The listing builds one solid part. Answer for the finished solid, in the listing's coordinates (mm). Face numbers are marked on the shaded views. A direction names the side the tool comes from. Give positions to 0.01 mm unless a question says otherwise; leave off trailing zeros. Order: outer loops, then holes, each group sorted by start corner. A loop starts at its lowest first (then second) coordinate and runs counter-clockwise, first axis right, second up. Notation, with made-up numbers: (-8.5, 35) - (6.5, 35) arc R34 ccw to (6.5, 66) - close; hole circle Ø3 at (37.25, 4.5). An arc over 180 degrees is marked (long way). Use a Markdown table: item, result. Add a question column.
1) Find section B-B, the plane z = 15. Determine the outline of the cut face in (x, y), plus the area to 3 significant figures.
2) For the marked faces 1 and 2, determine the directions among +Z, -Z, +X, -X, +Y, -Y from which every point of the face is accessible in a straight line to the end or side of a thin tool.
3) Find section C-C, the plane z = 0. Determine the outline of the cut face in (x, y), plus the area to 3 significant figures.
4) Find section D-D, the plane x = -2. Determine the outline of the cut face in (y, z).
5) Straight lines are drawn through the part: line 1 (X direction, y = 3.1, z = 0); line 2 (Z direction, x = -7, y = 3.55); line 3 (Y direction, x = -25, z = -9). For each, find the intervals that lie inside material, in ascending order.
6) The mould has two halves that part along X. Classify the marked faces 3 and 4: released by +X, released by -X, zero draft, split by the parting line, or undercut.
7) A flat-ended cylindrical pin translates along its axis: pin 1 (6 mm diameter, centred on x = 22.5, z = -0.5, fed in from +Y). Find the tip coordinate at first contact, or state that the pin passes through.
8) Find section A-A, the plane x = 15. Determine the outline of the cut face in (y, z), plus the area to 3 significant figures.
from build123d import *

# Parameters (mm, degrees)
CROQUIS1_W              = 70
CROQUIS1_H              = 40
SALIENTE_EXTRUIR1_DEPTH = 2
CROQUIS2_R              = 16
CROQUIS2_R_2            = 14
CROQUIS2_R_3            = 9.98
CROQUIS2_R_4            = 10
CROQUIS2_R_5            = 7.75
CROQUIS2_R_6            = 4.98
SALIENTE_EXTRUIR2_DEPTH = 2


with BuildPart() as part:
    # Croquis1 → Saliente-Extruir1 (new body)
    with BuildSketch(Plane(origin=(0, 0, 0), x_dir=(1, 0, 0), z_dir=(0, 1, 0))):
        Rectangle(CROQUIS1_W, CROQUIS1_H)
    extrude(amount=SALIENTE_EXTRUIR1_DEPTH)

    # Croquis2 → Saliente-Extruir2 (add)
    # profile 1 of 4: a face of its own
    with BuildSketch(Plane(origin=(0, 2, 0), x_dir=(1, 0, 0), z_dir=(0, 1, 0))):
        with Locations(Location((-15, 0, 0), (0, 0, 90))):
            Circle(CROQUIS2_R)
        with Locations(Location((-15, 0, 0), (0, 0, 270))):
            Circle(CROQUIS2_R_2, mode=Mode.SUBTRACT)
    # profile 2 of 4: a face of its own
    with BuildSketch(Plane(origin=(0, 2, 0), x_dir=(1, 0, 0), z_dir=(0, 1, 0))):
        with Locations(Location((-15, 0, 0), (0, 0, 90))):
            Circle(CROQUIS2_R_3)
    # profile 3 of 4: a face of its own
    with BuildSketch(Plane(origin=(0, 2, 0), x_dir=(1, 0, 0), z_dir=(0, 1, 0))):
        with Locations(Location((15, 0, 0), (0, 0, 90))):
            Circle(CROQUIS2_R_4)
        with Locations(Location((15, 0, 0), (0, 0, 270))):
            Circle(CROQUIS2_R_5, mode=Mode.SUBTRACT)
    # profile 4 of 4: a face of its own
    with BuildSketch(Plane(origin=(0, 2, 0), x_dir=(1, 0, 0), z_dir=(0, 1, 0))):
        with Locations(Location((15, 0, 0), (0, 0, 90))):
            Circle(CROQUIS2_R_6)
    extrude(amount=SALIENTE_EXTRUIR2_DEPTH)


solid = part.part
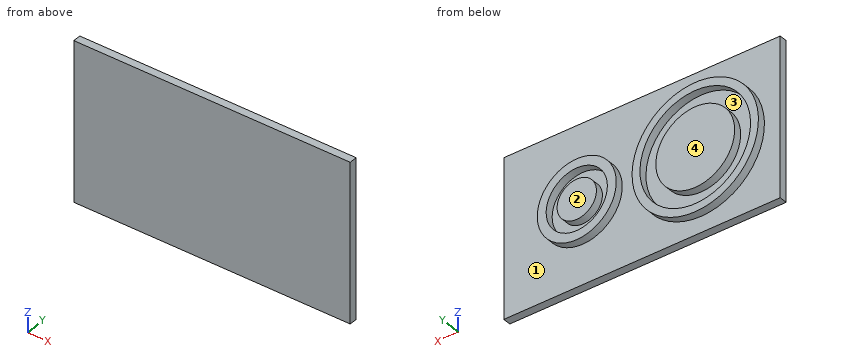
The answers:
| question | item | result |
|---|---|---|
| 1 | outline | (-35, 0) - (35, 0) - (35, 2) - (-9.43, 2) - (-9.43, 4) - (-20.57, 4) - (-20.57, 2) - (-35, 2) - close |
| 1 | area | 162 mm2 |
| 2 | face 1 | +Y |
| 2 | face 2 | +Z, -Z, +X, -X, +Y |
| 3 | outline | (-35, 0) - (35, 0) - (35, 2) - (25, 2) - (25, 4) - (22.75, 4) - (22.75, 2) - (19.98, 2) - (19.98, 4) - (10.02, 4) - (10.02, 2) - (7.25, 2) - (7.25, 4) - (5, 4) - (5, 2) - (1, 2) - (1, 4) - (-1, 4) - (-1, 2) - (-5.02, 2) - (-5.02, 4) - (-24.98, 4) - (-24.98, 2) - (-29, 2) - (-29, 4) - (-31, 4) - (-31, 2) - (-35, 2) - close |
| 3 | area | 217 mm2 |
| 4 | outline | (0, -20) - (2, -20) - (2, -9.33) - (4, -9.33) - (4, -5.2) - (2, -5.2) - (2, 5.2) - (4, 5.2) - (4, 9.33) - (2, 9.33) - (2, 20) - (0, 20) - close |
| 5 | line 1 | -31 to -29, -24.98 to -5.02, -1 to 1, 5 to 7.25, 10.02 to 19.98, 22.75 to 25 |
| 5 | line 2 | -13.86 to -11.49, -5.97 to 5.97, 11.49 to 13.86 |
| 5 | line 3 | 0 to 2 |
| 6 | face 3 | undercut |
| 6 | face 4 | zero draft |
| 7 | pin 1 | y = 4 |
| 8 | outline | (0, -20) - (2, -20) - (2, -10) - (4, -10) - (4, -7.75) - (2, -7.75) - (2, -4.98) - (4, -4.98) - (4, 4.98) - (2, 4.98) - (2, 7.75) - (4, 7.75) - (4, 10) - (2, 10) - (2, 20) - (0, 20) - close |
| 8 | area | 109 mm2 |
